from build123d import *

# Parameters (mm, degrees)
CROQUIS1_R              = 20
SALIENTE_EXTRUIR1_DEPTH = 0.4
CROQUIS3_R              = 0.35
CORTAR_EXTRUIR1_DEPTH   = 10
CROQUIS2_R              = 15
CROQUIS2_R_2            = 14
SALIENTE_EXTRUIR2_DEPTH = 0.5


with BuildPart() as part:
    # Croquis1 → Saliente-Extruir1 (new body)
    with BuildSketch(Plane.XY):
        Circle(CROQUIS1_R)
    extrude(amount=SALIENTE_EXTRUIR1_DEPTH)

    # Croquis3 → Cortar-Extruir1 (cut)
    with BuildSketch(Plane.XY.offset(0.4)):
        with Locations((12, 12)):
            Circle(CROQUIS3_R)
        with Locations((-12, 12)):
            Circle(CROQUIS3_R)
        with Locations((12, -12)):
            Circle(CROQUIS3_R)
        with Locations((-12, -12)):
            Circle(CROQUIS3_R)
    extrude(amount=-CORTAR_EXTRUIR1_DEPTH, mode=Mode.SUBTRACT)

    # Croquis2 → Saliente-Extruir2 (add)
    with BuildSketch(Plane.XY.offset(0.4)):
        Circle(CROQUIS2_R)
        Circle(CROQUIS2_R_2, mode=Mode.SUBTRACT)
    extrude(amount=SALIENTE_EXTRUIR2_DEPTH)


solid = part.part
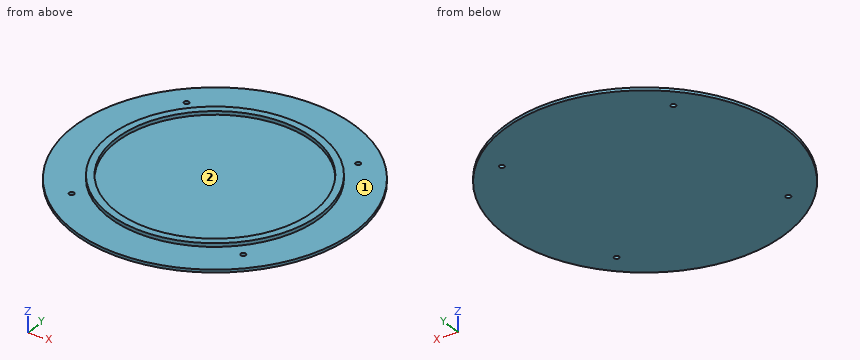
Input: part model. Units: mm. Frame: model coordinates. Face numbers are marked on the shaded views. Coordinates: 2 decimals unless noted, no trailing zeros. Loops run counter-clockwise (first coordinate to the right, second up) from the corner with the lowest first, then second, coordinate; pieces in that order, holes last. Notation, with made-up numbers: (43.5, -5.75) - (93.5, -5.75) arc R9 cw to (93.5, 7.25) - close; hole circle Ø3 at (-35, -11.5). An arc over 180 degrees is marked (long way). Answer in a Markdown table with one row per item. Add a question column.
Item 1: Section query A-A on z = 0.15. Return the cut outline in (x, y).
Item 2: Section query D-D on x = -14.5. Return the cut outline in (y, z).
Item 3: Line query: line 1 along Y through (x, z) = (0, 0.7); line 2 along Y through (x, z) = (-12, 0.15); line 3 along Z through (x, y) = (-5, -8). Output: solid intervals per line, ascending. Write a range as [from, to].
Item 4: Mould query, pull axis Y, two halves, no side actions, for the marked faces 1 and 2. Classes: released by +Y, released by -Y, zero draft, split by the parting line, or undercut.
Item 5: Contact query for a flat-ended pin moving along its axis: P1, Ø6, axis at x = -9, y = 1.5, coming from the +Z side. Output: stop coordinate, or through.
Item 6: Section query B-B on y = 0. Return the cut outline in (x, z), then the cut area to 3 significant figures.
Recorded:
| question | item | result |
|---|---|---|
| 1 | outline | circle Ø40 at (0, 0); hole circle Ø0.7 at (-12, -12); hole circle Ø0.7 at (-12, 12); hole circle Ø0.7 at (12, -12); hole circle Ø0.7 at (12, 12) |
| 2 | outline | (-13.77, 0) - (13.77, 0) - (13.77, 0.4) - (3.84, 0.4) - (3.84, 0.9) - (-3.84, 0.9) - (-3.84, 0.4) - (-13.77, 0.4) - close |
| 3 | line 1 | [-15, -14], [14, 15] |
| 3 | line 2 | [-16, -12.35], [-11.65, 11.65], [12.35, 16] |
| 3 | line 3 | [0, 0.4] |
| 4 | face 1 | zero draft |
| 4 | face 2 | undercut |
| 5 | P1 | z = 0.4 |
| 6 | outline | (-20, 0) - (20, 0) - (20, 0.4) - (15, 0.4) - (15, 0.9) - (14, 0.9) - (14, 0.4) - (-14, 0.4) - (-14, 0.9) - (-15, 0.9) - (-15, 0.4) - (-20, 0.4) - close |
| 6 | area | 17.0 mm^2 |
